```python
from build123d import *

# Parameters (mm, degrees)
F0_W      = 51
F0_H      = 55
F1_DEPTH  = 3
F2_W      = 51
F2_H      = 3
F3_DEPTH  = 15
F4_R      = 2.6
F4_R_2    = 1.6
F5_DEPTH  = 25
F6_R      = 2.1
F7_DEPTH  = 25
F9_DEPTH  = 25
F11_DEPTH = 25


with BuildPart() as f1:
    # F0 (on Top) → F1 (new body)
    with BuildSketch(Plane.XY):
        with Locations((25.5, 27.5)):
            Rectangle(F0_W, F0_H)
    extrude(amount=F1_DEPTH)

    # F2 (on face) → F3 (join)
    with BuildSketch(Plane.XY.offset(3)):
        with Locations((25.5, 1.5)):
            Rectangle(F2_W, F2_H)
    extrude(amount=F3_DEPTH)

    # F4 (on face) → F5 (cut)
    with BuildSketch(Plane.XZ):
        with Locations((7, 10)):
            Circle(F4_R)
        with Locations((29, 9)):
            Circle(F4_R_2)
    extrude(amount=-F5_DEPTH, mode=Mode.SUBTRACT)

    # F6 (on face) → F7 (cut)
    with BuildSketch(Plane.XY.offset(3)):
        with Locations((4, 10)):
            Circle(F6_R)
        with Locations((48, 47.788887)):
            Circle(F6_R)
    extrude(amount=-F7_DEPTH, mode=Mode.SUBTRACT)

    # F8 (on face) → F9 (cut)
    with BuildSketch(Plane.XY.offset(3)):
        Polygon((0, 15), (40, 55), (0, 55), align=None)
    extrude(amount=-F9_DEPTH, mode=Mode.SUBTRACT)

    # F10 (on face) → F11 (cut)
    with BuildSketch(Plane(origin=(0, 3, 0), x_dir=(-1, 0, 0), z_dir=(0, 1, 0))):
        Polygon((-51, 6), (-31, 18), (-51, 18), align=None)
    extrude(amount=-F11_DEPTH, mode=Mode.SUBTRACT)


solid = f1.part
```
Verification items for the finished model (mm, model axes). A direction names the side the tool comes from. Round coordinates to 2 decimals unless told otherwise and drop trailing zeros. Loops run counter-clockwise (first coordinate to the right, second up) from the corner with the lowest first, then second, coordinate; pieces in that order, holes last. Notation, with made-up numbers: (85, 6.25) -> (94, 6.25) arc R9 cw to (94, 16.25) -> close; hole circle Ø2 at (70.5, 47.25). An arc over 180 degrees is marked (long way). Answer as a JSON object with one key per item and string values.
Q1. Scan lines: line 1 (Z direction, x = 29, y = 1.75); line 2 (Y direction, x = 48, z = 1.25); line 3 (Z direction, x = 37.5, y = 29.5). Record each from-to range of solid material in increasing order. Write a range as from..to.
Data:
{"line 1": "z = 0..7.4, 10.6..18", "line 2": "y = 0..45.69, 49.89..55", "line 3": "z = 0..3"}
Q2. Draft check along X on faces 3 (the cylindrical face through (3.727, 12.082, 1.521)), 4 (the flat face through (0, 2, 5)), 5 (the flat face through (45, 55, 1)), 6 (the flat face through (41, 2, 12)). Enter one of: pulls with the +X half, pulls with the -X half, needs draft (parallel to the pull), parting line crosses it, or undercut.
Data:
{"face 3": "undercut", "face 4": "pulls with the -X half", "face 5": "needs draft", "face 6": "pulls with the +X half"}
Q3. Go/stop test with flat-tipped pins: P1, Ø12, axis at x = 19, y = 15, coming from the +Z side; P2, Ø3.5, axis at x = 29, z = 9, coming from the +Y side; P3, Ø6, axis at x = 18, z = 5.5, coming from the +Y side. Record where each tip stops, or that it passes through.
Data:
{"P1": "stops at z = 3", "P2": "stops at y = 3", "P3": "stops at y = 34.66"}
Q4. Section check A-A (z = 9). Record the boundary of the cut face in (x, y), then the cut area to 3 significant figures.
Data:
{"outline": "(0, 0) -> (4.6, 0) -> (4.6, 3) -> (0, 3) -> close; (9.4, 0) -> (27.4, 0) -> (27.4, 3) -> (9.4, 3) -> close; (30.6, 0) -> (46, 0) -> (46, 3) -> (30.6, 3) -> close", "area": "114 mm2"}
Q5. Section check D-D (y = 47). Record the boundary of the cut face in (x, z), then the cut area to 3 significant figures.
Data:
{"outline": "(32, 0) -> (46.05, 0) -> (46.05, 3) -> (32, 3) -> close; (49.95, 0) -> (51, 0) -> (51, 3) -> (49.95, 3) -> close", "area": "45.3 mm2"}
Q6. Section check C-C (x = 7). Record the boundary of the cut face in (y, z).
Data:
{"outline": "(0, 0) -> (22, 0) -> (22, 3) -> (3, 3) -> (3, 7.4) -> (0, 7.4) -> close; (0, 12.6) -> (3, 12.6) -> (3, 18) -> (0, 18) -> close"}
Q7. Section check B-B (x = 48). Record the boundary of the cut face in (y, z).
Data:
{"outline": "(0, 0) -> (45.69, 0) -> (45.69, 3) -> (3, 3) -> (3, 7.8) -> (0, 7.8) -> close; (49.89, 0) -> (55, 0) -> (55, 3) -> (49.89, 3) -> close"}
Q8. Access from +Z, -Z, +X, -X, +Y, -Y to the whole of each face (thin tool, end or side, straight path). Record for faces 1 (the flat face through (31, 24, 3)), 2 (the cylindrical face through (47.73, 49.87, 1.52)).
Data:
{"face 1": "+Z, +X, -X, +Y", "face 2": "+Z, -Z"}
